Geometry check sheet. Reference: the model listing, model coordinates, mm. A direction names the side the tool comes from. Give positions to 0.01 mm unless a question says otherwise; leave off trailing zeros. Order: outer loops, then holes, each group sorted by start corner. A loop starts at its lowest first (then second) coordinate and runs counter-clockwise, first axis right, second up. Notation, with made-up numbers: M 38.25,67 L 50.25,67 A13 cw 50.25,81 Z; hole C 67,65 d5. An arc over 180 degrees is marked long. Put each result on its own line as item: value. Start each with the question number.
Q1. Section check D-D on z = 54. Record the cut outline in (x, y).
Q2. Section check A-A on x = -20. Record the cut outline in (y, z), then the cut area to 3 significant figures.
Q3. Access from +Z, -Z, +X, -X, +Y, -Y to the whole of each face (thin tool, end or side, straight path). Record for faces 1 (the cylindrical face through (-56.056, -286.677, 42.103)), 2 (the flat face through (-25, -148, 8)).
Q4. Material ranges on L1, parallel to Y at x = -20, z = 2.25; L2, parallel to Y at x = -54.5, z = 34; L3, parallel to X at y = -230, z = 2, recorded low to high.
Q5. Section check B-B on y = -230. Record the cut outline in (x, z), then the cut area to 3 significant figures.
Q6. Mould release check, pull along Z, two halves, no side actions. Record for faces 3 (the cylindrical face through (-1.711, -147.9, 6.196)), 4 (the cylindrical face through (-20.91, -76.94, 3.94)), 5 (the cylindrical face through (-56.06, -14.84, 44.73)): +Z half, -Z half, draft (parallel to the pull), parting line (faces both ways), or undercut.
Q7. Section check C-C on y = -162. Record the cut outline in (x, z).
Q8. Go/stop test with flat-tipped pins: pin 1 (4 mm diameter, centred on y = -33.5, z = 37, fed in from +X); pin 2 (19 mm diameter, centred on x = -22, y = -110.5, fed in from +Z). Record where each tip stops, or that it passes through.
```python
from build123d import *

# Parameters (mm, degrees)
F1_DEPTH = 300
F2_R     = 7
F3_DEPTH = 25
F4_R     = 7
F5_DEPTH = 25


with BuildPart() as f1:
    # F0 (on Front) → F1 (new body)
    with BuildSketch(Plane.XZ):
        with BuildLine():
            Line((-60, 0), (0, 0))
            Line((0, 0), (0, 2))
            ThreePointArc((0, 2), (-1.757359, 6.242641), (-6, 8))
            Line((-6, 8), (-44, 8))
            ThreePointArc((-44, 8), (-49.656854, 10.343146), (-52, 16))
            Line((-52, 16), (-52, 74))
            ThreePointArc((-52, 74), (-53.757359, 78.242641), (-58, 80))
            Line((-58, 80), (-60, 80))
            Line((-60, 80), (-60, 0))
        make_face()
    extrude(amount=F1_DEPTH)

    # F2 (on face) → F3 (cut)
    with BuildSketch(Plane(origin=(-60, 0, 0), x_dir=(0, -1, 0), z_dir=(-1, 0, 0))):
        with Locations((20, 40)):
            Circle(F2_R)
        with Locations((150, 40)):
            Circle(F2_R)
        with Locations((280, 40)):
            Circle(F2_R)
    extrude(amount=-F3_DEPTH, mode=Mode.SUBTRACT)

    # F4 (on face) → F5 (cut)
    with BuildSketch(Plane(origin=(0, 0, 0), x_dir=(1, 0, 0), z_dir=(0, 0, -1))):
        with Locations((-20, 70)):
            Circle(F4_R)
        with Locations((-20, 230)):
            Circle(F4_R)
    extrude(amount=-F5_DEPTH, mode=Mode.SUBTRACT)


solid = f1.part
```
Results found:
1. outline: M -60,-300 L -52,-300 L -52,0 L -60,0 Z
2. outline: M -300,0 L -237,0 L -237,8 L -300,8 Z; M -223,0 L -77,0 L -77,8 L -223,8 Z; M -63,0 L 0,0 L 0,8 L -63,8 Z
2. area: 2,180 mm^2
3. face 1: +X, -X
3. face 2: +Z, +X, +Y, -Y
4. L1: y = -300 to -237, -223 to -77, -63 to 0
4. L2: y = -300 to -283.61, -276.39 to -153.61, -146.39 to -23.61, -16.39 to 0
4. L3: x = -60 to -27, -13 to 0
5. outline: M -60,0 L -27,0 L -27,8 L -44,8 A8 cw -52,16 L -52,74 A6 ccw -58,80 L -60,80 Z; M -13,0 L 0,0 L 0,2 A6 ccw -6,8 L -13,8 Z
5. area: 942 mm^2
6. face 3: +Z half
6. face 4: draft
6. face 5: undercut
7. outline: M -60,0 L 0,0 L 0,2 A6 ccw -6,8 L -44,8 A8 cw -52,16 L -52,74 A6 ccw -58,80 L -60,80 Z
8. pin 1: stops at x = -52
8. pin 2: stops at z = 8
